For this review, take the finished solid that the model builds, in its own axes (mm). A direction names the side the tool comes from. Round coordinates to 2 decimals unless told otherwise and drop trailing zeros. Write each loop counter-clockwise with the first axis right and the second up, starting at its lowest first coordinate (ties: lowest second). Pieces come first, ordered by that corner, then holes. Notation, with made-up numbers: M 19.25,41.25 L 66.25,41.25 A23 cw 66.25,54.25 Z; hole C 6,-20 d8. An arc over 180 degrees is marked long. Answer in a Markdown table with one row per item.
```python
from build123d import *

# Parameters (mm, degrees)
SKETCH1_W           = 38
SKETCH1_H           = 717
BOSS_EXTRUDE1_DEPTH = 190.5
SKETCH3_W           = 120
SKETCH3_H           = 25
BOSS_EXTRUDE2_DEPTH = 40
SKETCH4_R           = 10
CUT_EXTRUDE1_DEPTH  = 506
SKETCH5_R           = 15
BOSS_EXTRUDE3_DEPTH = 5


with BuildPart() as part:
    # Sketch1 → Boss-Extrude1 (new body)
    with BuildSketch(Plane(origin=(0, 0, 0), x_dir=(1, 0, 0), z_dir=(0, 1, 0))):
        with Locations((20.54028436, -361.58056872)):
            Rectangle(SKETCH1_W, SKETCH1_H)
    extrude(amount=BOSS_EXTRUDE1_DEPTH)

    # Sketch3 → Boss-Extrude2 (add)
    with BuildSketch(Plane.ZY.offset(-1.54028436)):
        with Locations((63.08056872, 158)):
            Rectangle(SKETCH3_W, SKETCH3_H)
        with Locations((63.08056872, 32.5)):
            Rectangle(SKETCH3_W, SKETCH3_H)
        with Locations((660.08056872, 32.5)):
            Rectangle(SKETCH3_W, SKETCH3_H)
        with Locations((660.08056872, 158)):
            Rectangle(SKETCH3_W, SKETCH3_H)
    extrude(amount=BOSS_EXTRUDE2_DEPTH)

    # Sketch4 → Cut-Extrude1 (cut)
    with BuildSketch(Plane(origin=(0, 170.5, 0), x_dir=(1, 0, 0), z_dir=(0, 1, 0))):
        with Locations((-18.45971564, -63.08056872)):
            Circle(SKETCH4_R)
        with Locations((-18.45971564, -660.08056872)):
            Circle(SKETCH4_R)
    extrude(amount=-CUT_EXTRUDE1_DEPTH, mode=Mode.SUBTRACT)

    # Sketch5 → Boss-Extrude3 (add)
    with BuildSketch(Plane.XZ):
        with Locations((20.54028436, 690.08056872)):
            Circle(SKETCH5_R)
        with Locations((20.54028436, 33.08056872)):
            Circle(SKETCH5_R)
    extrude(amount=BOSS_EXTRUDE3_DEPTH)


solid = part.part
```
Q1. Take a section at B-B (y = 33.5). State the section outline as (x, z) points, then the cut area to 3 significant figures.
Found:
| item | result |
|---|---|
| outline | M -38.46,3.08 L 39.54,3.08 L 39.54,720.08 L -38.46,720.08 L -38.46,600.08 L 1.54,600.08 L 1.54,123.08 L -38.46,123.08 Z; hole C -18.46,63.08 d20; hole C -18.46,660.08 d20 |
| area | 36,200 mm² |
Q2. For probe 1 along Z at (x, y) = (-10, 168.5); probe 2 along Z at (x, y) = (-4, 160); probe 3 along Z at (x, y) = (-22, 169), list the stretches that pass through material, from the lowest coordinate up.
Found:
| item | result |
|---|---|
| probe 1 | 3.08 to 57.75, 68.41 to 123.08, 600.08 to 654.75, 665.41 to 720.08 |
| probe 2 | 3.08 to 123.08, 600.08 to 720.08 |
| probe 3 | 3.08 to 53.73, 72.43 to 123.08, 600.08 to 650.73, 669.43 to 720.08 |
Q3. Insertion check: P1, Ø20, axis at x = -24, z = 644, coming from the +Y side; P2, Ø12, axis at x = 14.5, z = 548.5, coming from the -Y side; P3, Ø10, axis at y = 99, z = 371, coming from the -X side. Each pin has a flat end and moves straight along its axis. Give the tip position at first contact, or say it passes through.
Found:
| item | result |
|---|---|
| P1 | y = 170.5 |
| P2 | y = 0 |
| P3 | x = 1.54 |
Q4. Mouldability with a two-part tool opening along Y and no side actions: class faces 6 (the face through (-18, 20, 76)), 7 (the face through (-18, 145.5, 673)), 8 (the face through (-38.46, 158, 659)) as +Y half, -Y half, draft (parallel to the pull), parting line (faces both ways), or undercut.
Found:
| item | result |
|---|---|
| face 6 | -Y half |
| face 7 | undercut |
| face 8 | draft |
Q5. Take a section at D-D (y = 139). State the section outline as (x, z) points, then the cut area to 3 significant figures.
Found:
| item | result |
|---|---|
| outline | M 1.54,3.08 L 39.54,3.08 L 39.54,720.08 L 1.54,720.08 Z |
| area | 27,200 mm² |
Q6. Take a section at C-C (x = 16). State the section outline as (y, z) points.
Found:
| item | result |
|---|---|
| outline | M -5,18.78 L 0,18.78 L 0,3.08 L 190.5,3.08 L 190.5,720.08 L 0,720.08 L 0,704.38 L -5,704.38 L -5,675.78 L 0,675.78 L 0,47.38 L -5,47.38 Z |
Q7. Machinability: for faces 1 (the face through (-18, 20, 673)), 2 (the face through (-18, 170.5, 673)), 3 (the face through (-18, 45, 76)), 4 (the face through (-18, 32, 123.081)), 5 (the face through (19, -2, 48)), which of the approach directions +Z, -Z, +X, -X, +Y, -Y give a long, thin tool a straight path to every point of the face, cutting with its end or side? Answer none if there is none.
Found:
| item | result |
|---|---|
| face 1 | +Z, -Z, -X, -Y |
| face 2 | +Z, -Z, -X, +Y |
| face 3 | +Z, -Z, -X |
| face 4 | -X, +Y, -Y |
| face 5 | -Y |
Q8. Take a section at A-A (z = 622). State the section outline as (x, y) points.
Found:
| item | result |
|---|---|
| outline | M -38.46,20 L 1.54,20 L 1.54,0 L 39.54,0 L 39.54,190.5 L 1.54,190.5 L 1.54,170.5 L -38.46,170.5 L -38.46,145.5 L 1.54,145.5 L 1.54,45 L -38.46,45 Z |
